Can you work these out from the model? Positions are in its coordinate system, mm. A direction names the side the tool comes from. Give positions to 0.01 mm unless a question says otherwise; leave off trailing zeros. Loops run counter-clockwise (first coordinate to the right, second up) from the corner with the lowest first, then second, coordinate; pieces in that order, holes last. Notation, with made-up numbers: (18, 49.5) -> (57, 49.5) arc R8 cw to (57, 54.5) -> close; hole circle Ø1 at (81.25, -9.75). An arc over 180 degrees is marked (long way). One line per question, with ' | ' between items.
from build123d import *

# Parameters (mm, degrees)
BOSS_EXTRUDE1_DEPTH     = 4
CUT_EXTRUDE1_DEPTH      = 10
CUT_EXTRUDE1_DEPTH_BACK = 10
SKETCH2_R               = 5.75
BOSS_EXTRUDE5_DEPTH     = 58.68
SKETCH12_W              = 4
SKETCH12_H              = 61.717483032
BOSS_EXTRUDE8_DEPTH     = 50
SKETCH13_R              = 4
CUT_EXTRUDE5_DEPTH      = 20
SKETCH14_R              = 28.395
CUT_EXTRUDE6_DEPTH      = 10


with BuildPart() as part:
    # Sketch1 → Boss-Extrude1 (new body)
    with BuildSketch(Plane(origin=(0, 0, 0), x_dir=(1, 0, 0), z_dir=(0, 1, 0))):
        with BuildLine():
            Line((12.5, 0), (82.5, 0))
            ThreePointArc((82.5, 0), (91.338834765, 3.661165235), (95, 12.5))
            Line((95, 12.5), (95, 82.5))
            ThreePointArc((95, 82.5), (91.338834765, 91.338834765), (82.5, 95))
            Line((82.5, 95), (12.5, 95))
            ThreePointArc((12.5, 95), (3.661165235, 91.338834765), (0, 82.5))
            Line((0, 82.5), (0, 12.5))
            ThreePointArc((0, 12.5), (3.661165235, 3.661165235), (12.5, 0))
        make_face()
    extrude(amount=BOSS_EXTRUDE1_DEPTH)

    # Sketch2 → Cut-Extrude1 (cut, two sides: drawn at the far end of the back side and taken through both)
    with BuildSketch(Plane(origin=(0, 4, 0), x_dir=(1, 0, 0), z_dir=(0, 1, 0)).offset(-CUT_EXTRUDE1_DEPTH_BACK)):
        with Locations(Location((12.5, 82.5, 0), (0, 0, 90))):
            Circle(SKETCH2_R)
        with Locations(Location((82.5, 82.5, 0), (0, 0, 90))):
            Circle(SKETCH2_R)
        with Locations(Location((12.5, 12.5, 0), (0, 0, 90))):
            Circle(SKETCH2_R)
        with Locations(Location((82.5, 12.5, 0), (0, 0, 90))):
            Circle(SKETCH2_R)
    extrude(amount=CUT_EXTRUDE1_DEPTH + CUT_EXTRUDE1_DEPTH_BACK, mode=Mode.SUBTRACT)

    # Sketch8 → Boss-Extrude5 (add)
    with BuildSketch(Plane.ZY):
        Polygon((-17.641258484, 4), (-16.641258484, 4), (-16.641258484, 0), (-78.358741516, 0), (-78.358741516, 4), (-77.358741516, 4), align=None)
    extrude(amount=BOSS_EXTRUDE5_DEPTH)

    # Sketch12 → Boss-Extrude8 (add)
    with BuildSketch(Plane(origin=(0, 4, 0), x_dir=(1, 0, 0), z_dir=(0, 1, 0))):
        with Locations((-56.68, 47.5)):
            Rectangle(SKETCH12_W, SKETCH12_H)
    extrude(amount=BOSS_EXTRUDE8_DEPTH)

    # Sketch13 → Cut-Extrude5 (cut)
    with BuildSketch(Plane.ZY.offset(58.68)):
        with Locations((-66.858741516, 44)):
            Circle(SKETCH13_R)
        with Locations((-26.641258484, 44)):
            Circle(SKETCH13_R)
    extrude(amount=-CUT_EXTRUDE5_DEPTH, mode=Mode.SUBTRACT)

    # Sketch14 → Cut-Extrude6 (cut)
    with BuildSketch(Plane(origin=(0, 4, 0), x_dir=(1, 0, 0), z_dir=(0, 1, 0))):
        with Locations(Location((47.5, 47.5, 0), (0, 0, 270))):
            Circle(SKETCH14_R)
    extrude(amount=-CUT_EXTRUDE6_DEPTH, mode=Mode.SUBTRACT)


solid = part.part
Q1. On a 3-axis mill with a long thin cutter (end or side, diameter ignored), from which of +Z, -Z, +X, -X, +Y, -Y can I reach the whole of each face in a straight line? I mean faces 1 (the face through (-43, 3, -16.641)), 2 (the face through (-57, 54, -48)), 3 (the face through (0, 2, -80)). Say none if no direction works.
Entries:
face 1: +Z, -X, +Y, -Y | face 2: +Z, -Z, +X, -X, +Y | face 3: -Z, -X, +Y, -Y
Q2. If we section it at C-C (z = -29): Write out the boundary of the cut face in (x, y).
Entries:
outline: (-58.68, 0) -> (25.96, 0) -> (25.96, 4) -> (-54.68, 4) -> (-54.68, 40.77) -> (-58.68, 40.77) -> close; (-58.68, 47.23) -> (-54.68, 47.23) -> (-54.68, 54) -> (-58.68, 54) -> close; (69.04, 0) -> (95, 0) -> (95, 4) -> (69.04, 4) -> close
Q3. If we section it at B-B (x = 79): Write out the boundary of the cut face in (y, z), plus the area to 3 significant figures.
Entries:
outline: (0, -95) -> (4, -95) -> (4, -87.06) -> (0, -87.06) -> close; (0, -77.94) -> (4, -77.94) -> (4, -17.06) -> (0, -17.06) -> close; (0, -7.94) -> (4, -7.94) -> (4, 0) -> (0, 0) -> close | area: 307 mm²
Q4. If we mould it in two halves opening along X, with no side actions, what happens to faces 4 (the face through (19, 4, -38)), 5 (the face through (12.247, 1.972, -76.756)), 6 (the face through (0, 2, -15))? For each: pulls with the +X half, pulls with the -X half, needs draft (parallel to the pull), parting line crosses it, or undercut.
Entries:
face 4: needs draft | face 5: undercut | face 6: pulls with the -X half
Q5. If I drill on probe 1 along X at (y, z) = (2, -82); probe 2 along X at (y, z) = (2.35, -47.5) (3 decimals); probe 3 along Y at (x, z) = (51, -84), over which ranges is the centre line in solid material (lowest first)? Write a range as from..to.
Entries:
probe 1: 0..6.77, 18.23..76.77, 88.23..95 | probe 2: -58.68..19.105, 75.895..95 | probe 3: 0..4
Q6. If we section it at A-A (x = 47.5): Write out the boundary of the cut face in (y, z) (3 decimals), plus the area to 3 significant figures.
Entries:
outline: (0, -95) -> (4, -95) -> (4, -75.895) -> (0, -75.895) -> close; (0, -19.105) -> (4, -19.105) -> (4, 0) -> (0, 0) -> close | area: 153 mm²
Q7. For pin 1 Ø9 at (y, z) = (44, -66.86) entering from +X; pin 2 Ø15 at (x, z) = (82.5, -82.5) entering from +Y; pin 3 Ø1.2 at (y, z) = (1.5, -80) entering from -X, each with a flat end and sliding along its axis, tell me the tip position at first contact or that it passes through.
Entries:
pin 1: x = -54.68 | pin 2: y = 4 | pin 3: x = 0
Q8. If we section it at D-D (z = -55): Write out the boundary of the cut face in (x, y).
Entries:
outline: (-58.68, 0) -> (20.11, 0) -> (20.11, 4) -> (-54.68, 4) -> (-54.68, 54) -> (-58.68, 54) -> close; (74.89, 0) -> (95, 0) -> (95, 4) -> (74.89, 4) -> close
